from build123d import *

# Parameters (mm, degrees)
F1_DEPTH     = 15
F3_DEPTH     = 6
F5_DEPTH     = 18
F6_R         = 10
F9_DEPTH     = 6
F10_DEPTH    = 6
F11_R        = 2
F13_DEPTH    = 6
F15_R        = 10
F19_DEPTH    = 50.001
F21_DEPTH    = 45.001
F23_DEPTH    = 6
F24_T1_DEPTH = 6


# Not quite as in the source:
# - a fillet or chamfer that OpenCascade refuses, or shapes differently, is made with other operations: its cross-section is extruded or revolved along the edge and cut away or added


with BuildPart() as f1:
    # F0 (on Front) → F1 (new body, symmetric)
    with BuildSketch(Plane.XZ):
        Polygon((9, -17.5), (9, 17.5), (3, 17.5), (3, 27.5), (-3, 27.5), (-3, 17.5), (-9, 17.5), (-9, -17.5), (-9, -27.5), (-3, -27.5), (-3, -17.5), (3, -17.5), (3, -27.5), (9, -27.5), align=None)
    extrude(amount=F1_DEPTH, both=True)

    # F2 (on face) → F3 (cut)
    with BuildSketch(Plane(origin=(-3, 0, 0), x_dir=(0, -1, 0), z_dir=(-1, 0, 0))):
        with BuildLine():
            ThreePointArc((0, 25.12), (-2.62, 22.5), (0, 19.88))
            Line((0, 19.88), (0, 25.12))
        make_face()
        with BuildLine():
            Line((0, 25.12), (0, 19.88))
            ThreePointArc((0, 19.88), (1.8526197667, 20.6473802333), (2.62, 22.5))
            ThreePointArc((2.62, 22.5), (1.8526197667, 24.3526197667), (0, 25.12))
        make_face()
    extrude(amount=-F3_DEPTH, mode=Mode.SUBTRACT)

    # F4 (on face) → F5 (cut)
    with BuildSketch(Plane(origin=(-9, 0, 0), x_dir=(0, -1, 0), z_dir=(-1, 0, 0))):
        with BuildLine():
            ThreePointArc((0, -25.12), (1.8526197667, -24.3526197667), (2.62, -22.5))
            ThreePointArc((2.62, -22.5), (-1.8526197667, -20.6473802333), (0, -25.12))
        make_face()
    extrude(amount=-F5_DEPTH, mode=Mode.SUBTRACT)

    # F6
    f6_edges = [f1.edges().sort_by_distance(p)[0] for p in [
        (0, 15, 27.5),
        (0, -15, 27.5),
        (6, -15, -27.5),
        (-6, -15, -27.5),
    ]]
    fillet(f6_edges, radius=F6_R)

    # F8 (on face) → F9 (cut)
    with BuildSketch(Plane(origin=(-9, 0, 0), x_dir=(0, -1, 0), z_dir=(-1, 0, 0))):
        with BuildLine():
            ThreePointArc((-7, 16.0872004348), (-5.1915204429, 10.3514360713), (-0.4202014333, 6.690274227))
            Line((-0.4202014333, 6.690274227), (15, 1.0777798989))
            Line((15, 1.0777798989), (15, 17.5))
            Line((15, 17.5), (-7, 17.5))
            Line((-7, 17.5), (-7, 16.0872004348))
        make_face()
    extrude(amount=-F9_DEPTH, mode=Mode.SUBTRACT)

    # F7 (on face) → F10 (cut)
    with BuildSketch(Plane.YZ.offset(9)):
        with BuildLine():
            Line((7, 17.5), (-15, 17.5))
            Line((-15, 17.5), (-15, 1.07778))
            Line((-15, 1.07778), (0.4202014333, 6.6902743281))
            ThreePointArc((0.4202014333, 6.6902743281), (5.1915204429, 10.3514361724), (7, 16.087200536))
            Line((7, 16.087200536), (7, 17.5))
        make_face()
    extrude(amount=-F10_DEPTH, mode=Mode.SUBTRACT)

    # F11
    f11_edges = [f1.edges().sort_by_distance(p)[0] for p in [
        (9, 15, -5),
        (-9, 15, -5),
    ]]
    fillet(f11_edges, radius=F11_R)

    # F12 (on face) → F13 (cut)
    with BuildSketch(Plane(origin=(-3, 0, 0), x_dir=(0, -1, 0), z_dir=(-1, 0, 0))):
        with BuildLine():
            Line((5, 27.5), (0, 27.5))
            ThreePointArc((0, 27.5), (3.5355339059, 26.0355339059), (5, 22.5))
            Line((5, 22.5), (5, 4.7174822415))
            Line((5, 4.7174822415), (15, 1.0777798989))
            Line((15, 1.0777798989), (15, 17.5))
            ThreePointArc((15, 17.5), (12.0710678119, 24.5710678119), (5, 27.5))
        make_face()
    extrude(amount=-F13_DEPTH, mode=Mode.SUBTRACT)

    # F15
    f15_edges = [f1.edges().sort_by_distance(p)[0] for p in [
        (0, -15, -17.5),
    ]]
    fillet(f15_edges, radius=F15_R)

    # F18 (on face) → F19 (cut, through all)
    with BuildSketch(Plane.XY.offset(22.5)):
        with BuildLine():
            ThreePointArc((2, -10), (1.4142135624, -8.5857864376), (0, -8))
            Line((0, -8), (0, -12))
            ThreePointArc((0, -12), (1.4142135624, -11.4142135624), (2, -10))
        make_face()
        with BuildLine():
            Line((0, -12), (0, -8))
            ThreePointArc((0, -8), (-2, -10), (0, -12))
        make_face()
    extrude(amount=-F19_DEPTH, mode=Mode.SUBTRACT)

    # F20 (on face) → F21 (cut, through all)
    with BuildSketch(Plane(origin=(0, 0, -17.5), x_dir=(1, 0, 0), z_dir=(0, 0, -1))):
        with BuildLine():
            ThreePointArc((0, -9), (-2, -11), (0, -13))
            Line((0, -13), (0, -11))
            Line((0, -11), (0, -9))
        make_face()
        with BuildLine():
            Line((0, -11), (0, -13))
            ThreePointArc((0, -13), (1.4142135624, -12.4142135624), (2, -11))
            ThreePointArc((2, -11), (1.4142135624, -9.5857864376), (0, -9))
            Line((0, -9), (0, -11))
        make_face()
    extrude(amount=-F21_DEPTH, mode=Mode.SUBTRACT)

    # F22 (on face) → F23 (cut)
    with BuildSketch(Plane.YZ.offset(3)):
        with BuildLine():
            ThreePointArc((0, 17.5), (-3.5355339059, 18.9644660941), (-5, 22.5))
            Line((-5, 22.5), (-5, 4.7174822415))
            Line((-5, 4.7174822415), (0, 6.5373334129))
            Line((0, 6.5373334129), (0, 17.5))
        make_face()
    extrude(amount=-F23_DEPTH, mode=Mode.SUBTRACT)

    # F24: fillet of radius 5 on 2 edges, made by hand

    # F24_s2 → F24_t1 (join)
    with BuildSketch(Plane.YZ.offset(-3)):
        with BuildLine():
            ThreePointArc((-2.5, 18.1698729811), (-0.6698729811, 16.3397459622), (0, 13.8397459622))
            Line((0, 13.8397459622), (0, 17.5))
            ThreePointArc((0, 17.5), (-1.2940952255, 17.6703708686), (-2.5, 18.1698729811))
        make_face()
        with BuildLine():
            ThreePointArc((-3.2898992834, 5.3399081011), (-0.9042397786, 7.1704890233), (0, 10.038371205))
            Line((0, 10.038371205), (0, 6.5373334129))
            Line((0, 6.5373334129), (-3.2898992834, 5.3399081011))
        make_face()
    extrude(amount=F24_T1_DEPTH)


solid = f1.part
Model file for the job. Use its own axes, mm. A direction names the side the tool comes from. Round coordinates to 2 decimals unless told otherwise and drop trailing zeros. Order: outer loops, then holes, each group sorted by start corner. A loop starts at its lowest first (then second) coordinate and runs counter-clockwise, first axis right, second up. Notation, with made-up numbers: M 16.5,52 L 67.5,52 A24 cw 67.5,64 Z; hole C -38,73 d9. An arc over 180 degrees is marked long. Write each question's results on one line, items separated by ' | '. Start each with the question number.
(1) Drop flat-ended pins along their axis: pin 1 (5 mm diameter, centred on x = -6, y = 9, fed in from +Z); pin 2 (4 mm diameter, centred on x = 0, y = 7, fed in from -Z); pin 3 (1.1 mm diameter, centred on x = -7.5, z = 17, fed in from -Y). Give the stop position or say it passes through.
(2) Probe probe 1 along X at (y, z) = (7, -21); probe 2 along Y at (x, z) = (-1, -10.5); probe 3 along X at (y, z) = (11, -14.5). List the from-to ranges inside material, lowest first. Write a range as from..to.
(3) Two-plate mould, pull along X, no slides. Class faces 1 (the face through (9, -1, -10)), 2 (the face through (0.042, -13.128, -13.325)), 3 (the face through (-6, 7, 17)): pulls with the +X half, pulls with the -X half, needs draft (parallel to the pull), parting line crosses it, or undercut.
(4) Saw through at C-C, the plane z = 11. Give the cut face in (x, y), then the cut area to 3 significant figures.
(5) Saw through at A-A, the plane z = 21. Give the cut face in (x, y).
(6) Which spindle directions (+Z, -Z, +X, -X, +Y, -Y) get a long thin tool onto all of the face, cutting with end or side? Do faces 4 (the face through (-0.042, -0.929, 7.136)), 5 (the face through (3, -0.2, -19.6)), 6 (the face through (-6.04, 5.24, 10.42)). Say none if no direction does.
(7) Saw through at B-B, the plane z = 0. Give the cut face in (x, y).
Established:
1) pin 1: stops at z = 17.5 | pin 2: stops at z = -17.5 | pin 3: stops at y = 7
2) probe 1: x = -9..-3, 3..9 | probe 2: y = -14.54..-11.73, -8.27..9.27, 12.73..15 | probe 3: x = -9..-2, 2..9
3) face 1: pulls with the +X half | face 2: undercut | face 3: needs draft
4) outline: M -9,5.61 L -3,5.61 L -3,0 L 3,0 L 3,5.61 L 9,5.61 L 9,13 A2 ccw 7,15 L -7,15 A2 ccw -9,13 Z; hole C 0,11 d4 | area: 188 mm^2
5) outline: M -3,-4.77 L 3,-4.77 L 3,-2.15 L -3,-2.15 Z; M -3,2.15 L 3,2.15 L 3,14.37 L -3,14.37 Z; hole C 0,11 d4
6) face 4: +X, -X, -Y | face 5: -Z, -Y | face 6: +Z, -X, -Y
7) outline: M -9,-15 L 9,-15 L 9,13 A2 ccw 7,15 L -7,15 A2 ccw -9,13 Z; hole C 0,-10 d4; hole C 0,11 d4
